Can you work these out from the drawing? Everything is in mm from the part's minimum corner. A direction names the side the tool comes from. Coordinates: 2 decimals unless noted, no trailing zeros. Order: outer loops, then holes, each group sorted by start corner. A loop starts at its lowest first (then second) coordinate and runs counter-clockwise, first axis right, second up. Notation, with made-up numbers: (5.25, 36.25) -> (44.25, 36.25) arc R28 ccw to (44.25, 71.25) -> close; hole circle Ø1 at (29, 26). An arc over 180 degrees is marked (long way). Use a Markdown table: item, result. Add a question column.
1) Will these pins go through, and if not, where does the flat tip stop? pin 1 Ø4 at (x, z) = (46, 21) entering from -Y; pin 2 Ø3 at (x, z) = (30.5, 12) entering from +Y.
2) If we section it at D-D (y = 4): Write out the boundary of the cut face in (x, z).
3) If we section it at A-A (x = 11.5): Write out the boundary of the cut face in (y, z), plus the area to 3 significant figures.
4) If we section it at B-B (z = 12.5): Write out the boundary of the cut face in (x, y).
5) Which directions (+Z, -Z, +X, -X, +Y, -Y) give clear straight access to the entire face, cutting with the end or side of a thin tool? Please do the marked faces 5 and 6.
6) If we section it at C-C (x = 4): Write out the boundary of the cut face in (y, z).
7) Thinking about a two-plate mould opening in Z: for the marked faces 1, 2, 3 and 4, which applies, +Z half, -Z half, draft (parallel to the pull), parting line (faces both ways), or undercut?
8) If I drill on L1, parallel to Z at x = 40, y = 7.25; L2, parallel to Z at x = 46, y = 0.6; L3, parallel to Z at x = 11.5, y = 1.1, over which ranges is the centre line in solid material (lowest first)? Write a range as [from, to].
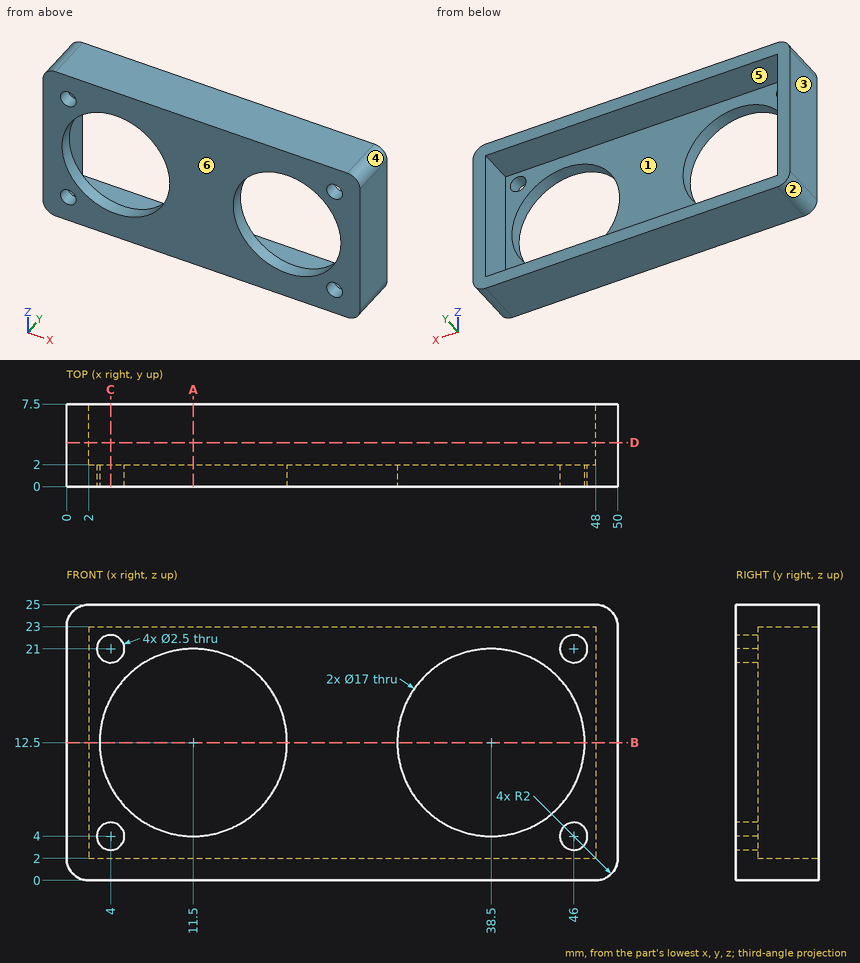
Answer sheet:
| question | item | result |
|---|---|---|
| 1 | pin 1 | y = 0 |
| 1 | pin 2 | y = 2 |
| 2 | outline | (0, 2) arc R2 ccw to (2, 0) -> (48, 0) arc R2 ccw to (50, 2) -> (50, 23) arc R2 ccw to (48, 25) -> (2, 25) arc R2 ccw to (0, 23) -> close; hole (2, 2) -> (48, 2) -> (48, 23) -> (2, 23) -> close |
| 3 | outline | (0, 0) -> (7.5, 0) -> (7.5, 2) -> (2, 2) -> (2, 4) -> (0, 4) -> close; (0, 21) -> (2, 21) -> (2, 23) -> (7.5, 23) -> (7.5, 25) -> (0, 25) -> close |
| 3 | area | 38.0 mm2 |
| 4 | outline | (0, 0) -> (3, 0) -> (3, 2) -> (2, 2) -> (2, 7.5) -> (0, 7.5) -> close; (20, 0) -> (30, 0) -> (30, 2) -> (20, 2) -> close; (47, 0) -> (50, 0) -> (50, 7.5) -> (48, 7.5) -> (48, 2) -> (47, 2) -> close |
| 5 | face 5 | +Y |
| 5 | face 6 | +Z, -Z, +X, -X, -Y |
| 6 | outline | (0, 0) -> (7.5, 0) -> (7.5, 2) -> (2, 2) -> (2, 2.75) -> (0, 2.75) -> close; (0, 5.25) -> (2, 5.25) -> (2, 8.5) -> (0, 8.5) -> close; (0, 16.5) -> (2, 16.5) -> (2, 19.75) -> (0, 19.75) -> close; (0, 22.25) -> (2, 22.25) -> (2, 23) -> (7.5, 23) -> (7.5, 25) -> (0, 25) -> close |
| 7 | face 1 | undercut |
| 7 | face 2 | -Z half |
| 7 | face 3 | draft |
| 7 | face 4 | +Z half |
| 8 | L1 | [0, 2], [23, 25] |
| 8 | L2 | [0, 2.75], [5.25, 8.5], [16.5, 19.75], [22.25, 25] |
| 8 | L3 | [0, 4], [21, 25] |
